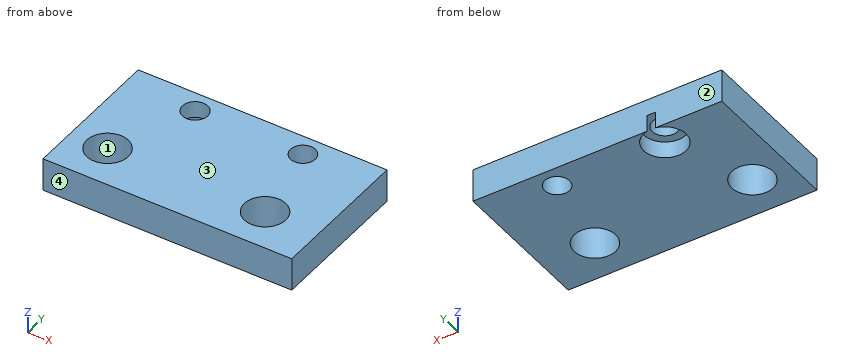
```python
from build123d import *

# Parameters (mm, degrees)
ESQUISSE2_W             = 60
ESQUISSE2_H             = 35
BASE_EXTRUSION_DEPTH    = 8
ESQUISSE4_R             = 3.05
ESQUISSE4_R_2           = 3
ESQUISSE4_R_3           = 5
ENL_V_MAT_EXTRU_1_DEPTH = 8
ESQUISSE5_R             = 5.1
ENL_V_MAT_EXTRU_2_DEPTH = 4


with BuildPart() as part:
    # Esquisse2 → Base-Extrusion (new body)
    with BuildSketch(Plane.XY):
        with Locations((0, 7.5)):
            Rectangle(ESQUISSE2_W, ESQUISSE2_H)
    extrude(amount=BASE_EXTRUSION_DEPTH)

    # Esquisse4 → Enlèv. mat.-Extru.1 (cut)
    with BuildSketch(Plane.XY.offset(8)):
        with Locations((-13, 20)):
            Circle(ESQUISSE4_R)
        with Locations((13, 20)):
            Circle(ESQUISSE4_R_2)
        with Locations((-21, 0)):
            Circle(ESQUISSE4_R_3)
        with Locations((17, 0)):
            Circle(ESQUISSE4_R_3)
    extrude(amount=-ENL_V_MAT_EXTRU_1_DEPTH, mode=Mode.SUBTRACT)

    # Esquisse5 → Enlèv. mat.-Extru.2 (cut)
    with BuildSketch(Plane(origin=(0, 0, 0), x_dir=(-1, 0, 0), z_dir=(0, 0, -1))):
        with Locations((13, 20)):
            Circle(ESQUISSE5_R)
    extrude(amount=-ENL_V_MAT_EXTRU_2_DEPTH, mode=Mode.SUBTRACT)


solid = part.part
```
Check sheet for the modelled part. Datum: model origin and axes. Units: mm. Face numbers are marked on the shaded views. Round coordinates to 2 decimals unless told otherwise and drop trailing zeros. Write each loop counter-clockwise with the first axis right and the second up, starting at its lowest first coordinate (ties: lowest second). Pieces come first, ordered by that corner, then holes. Notation, with made-up numbers: M -27.5,-4.5 L -12.5,-4.5 A13 ccw -12.5,11.5 Z; hole C 49.25,43.25 d9. An arc over 180 degrees is marked long. Write item = value, one per line. Start each with the question number.
1. Section check D-D, the plane x = -21. Record the cut outline in (y, z).
2. Scan lines: line 1 (Y direction, x = -13, z = 6.3); line 2 (X direction, y = 1, z = 3); line 3 (X direction, y = 22.5, z = 2.5). Record each from-to range of solid material in increasing order. Write a range as [from, to].
3. Section check B-B, the plane x = 13. Record the cut outline in (y, z), then the cut area to 3 significant figures.
4. Section check C-C, the plane y = 0. Record the cut outline in (x, z).
5. Release check for a two-part mould opening along Y. For the marked faces 1, 2, 3 and 4 record: pulls with the +Y half, pulls with the -Y half, needs draft (parallel to the pull), parting line crosses it, or undercut.
6. Gauge pin test, flat end, axial feed: pin 1 (5 mm diameter, centred on x = -14, y = 19, fed in from -Z). Record the tip position at first contact, or that the pin passes through.
7. Section check A-A, the plane z = 6. Record the cut outline in (x, y), then the cut area to 3 significant figures.
Results found:
q1.outline = M -10,0 L -5,0 L -5,8 L -10,8 Z; M 5,0 L 25,0 L 25,8 L 5,8 Z
q2.line_1 = [-10, 16.95], [23.05, 25]
q2.line_2 = [-30, -25.9], [-16.1, 12.1], [21.9, 30]
q2.line_3 = [-30, -17.45], [-8.55, 11.34], [14.66, 30]
q3.outline = M -10,0 L -3,0 L -3,8 L -10,8 Z; M 3,0 L 17,0 L 17,8 L 3,8 Z; M 23,0 L 25,0 L 25,8 L 23,8 Z
q3.area = 184 mm^2
q4.outline = M -30,0 L -26,0 L -26,8 L -30,8 Z; M -16,0 L 12,0 L 12,8 L -16,8 Z; M 22,0 L 30,0 L 30,8 L 22,8 Z
q5.face_1 = undercut
q5.face_2 = pulls with the +Y half
q5.face_3 = needs draft
q5.face_4 = pulls with the -Y half
q6.pin_1 = 4
q7.outline = M -30,-10 L 30,-10 L 30,25 L -30,25 Z; hole C -21,0 d10; hole C -13,20 d6.1; hole C 13,20 d6; hole C 17,0 d10
q7.area = 1,890 mm^2
